Here's the drawing with two shaded views (mm, measured from the low corner). I have some questions. A direction names the side the tool comes from. Coordinates: 2 decimals unless noted, no trailing zeros. Write each loop counter-clockwise with the first axis right and the second up, starting at its lowest first coordinate (ties: lowest second). Pieces come first, ordered by that corner, then holes.
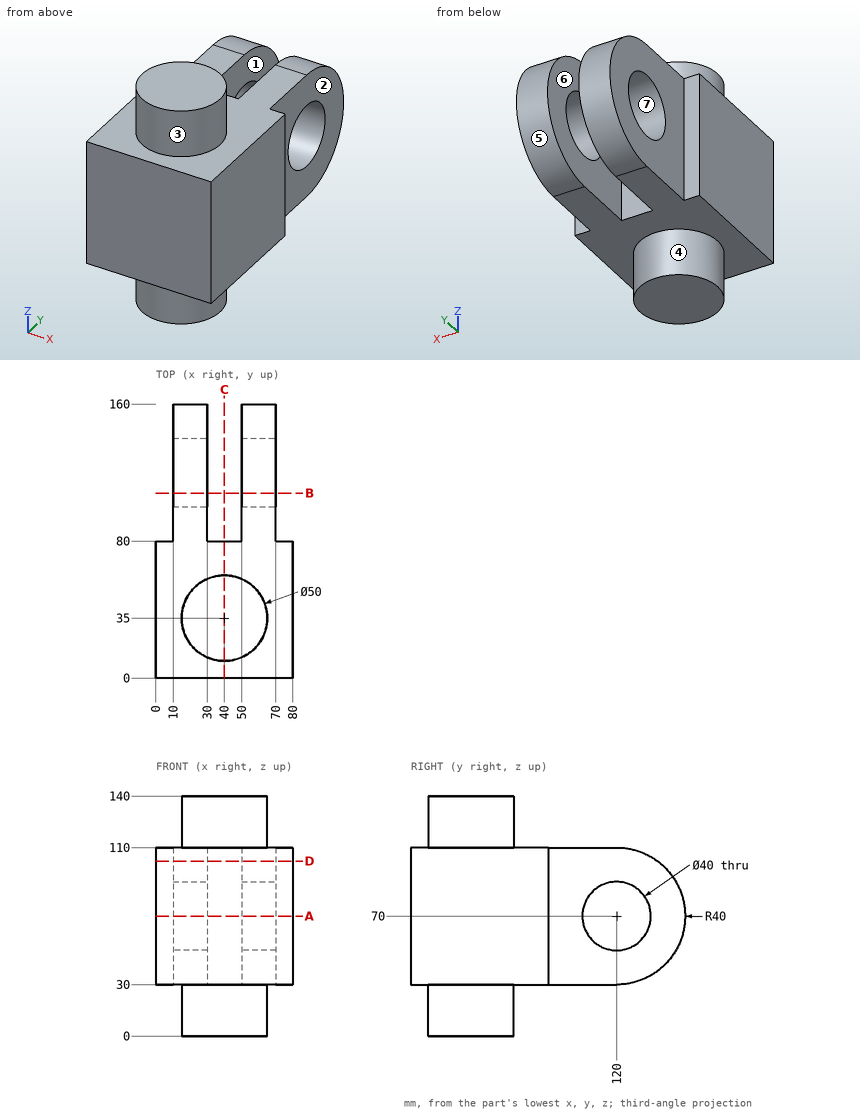
1. If I drill on L1, parallel to Y at x = 16, z = 70; L2, parallel to X at y = 138, z = 48.5; L3, parallel to Y at x = 48, z = 77.5, over which ranges is the centre line in solid material (lowest first)?
2. Which directions (+Z, -Z, +X, -X, +Y, -Y) give clear straight access to the entire face, cutting with the end or side of a thin tool? Please do the marked faces 1, 2, 3 and 4.
3. If we section it at A-A, the plane z = 70: List the corners of the cut face in (x, y) for me.
4. If we section it at D-D, the plane z = 102: List the corners of the cut face in (x, y) for me.
5. We'd pull the mould along Z, two halves only. Please class the marked faces 5, 6 and 7: released by +Z, released by -Z, zero draft, split by the parting line, or undercut.
6. If we section it at C-C, the plane x = 40: List the corners of the cut face in (y, z) for me.
7. If we section it at B-B, the plane y = 108: List the corners of the cut face in (x, z) for me.
8. I'm going to push flat-ended pins straight in: P1, Ø3, axis at x = 76.5, z = 68, coming from the +Y side; P2, Ø22, axis at x = 40.5, z = 86.5, coming from the +Y side; P3, Ø24, axis at y = 128, z = 82, coming from the -X side; P4, Ø1.5, axis at x = 31.5, y = 141, coming from the -Z side. Where does each tip first touch, or does it pass through?
Answers:
1. L1: y = 0 to 100, 140 to 160
1. L2: x = 10 to 30, 50 to 70
1. L3: y = 0 to 80
2. face 1: +Z, -Z, +Y
2. face 2: +Z, -Z, +X, +Y
2. face 3: +Z
2. face 4: -Z
3. outline: (0, 0) - (80, 0) - (80, 80) - (70, 80) - (70, 100) - (50, 100) - (50, 80) - (30, 80) - (30, 100) - (10, 100) - (10, 80) - (0, 80) - close; (10, 140) - (30, 140) - (30, 160) - (10, 160) - close; (50, 140) - (70, 140) - (70, 160) - (50, 160) - close
4. outline: (0, 0) - (80, 0) - (80, 80) - (70, 80) - (70, 144) - (50, 144) - (50, 80) - (30, 80) - (30, 144) - (10, 144) - (10, 80) - (0, 80) - close
5. face 5: split by the parting line
5. face 6: zero draft
5. face 7: undercut
6. outline: (0, 30) - (10, 30) - (10, 0) - (60, 0) - (60, 30) - (80, 30) - (80, 110) - (60, 110) - (60, 140) - (10, 140) - (10, 110) - (0, 110) - close
7. outline: (10, 30) - (30, 30) - (30, 54) - (10, 54) - close; (10, 86) - (30, 86) - (30, 110) - (10, 110) - close; (50, 30) - (70, 30) - (70, 54) - (50, 54) - close; (50, 86) - (70, 86) - (70, 110) - (50, 110) - close
8. P1: stops at y = 80
8. P2: stops at y = 158.47
8. P3: stops at x = 10
8. P4: passes through
